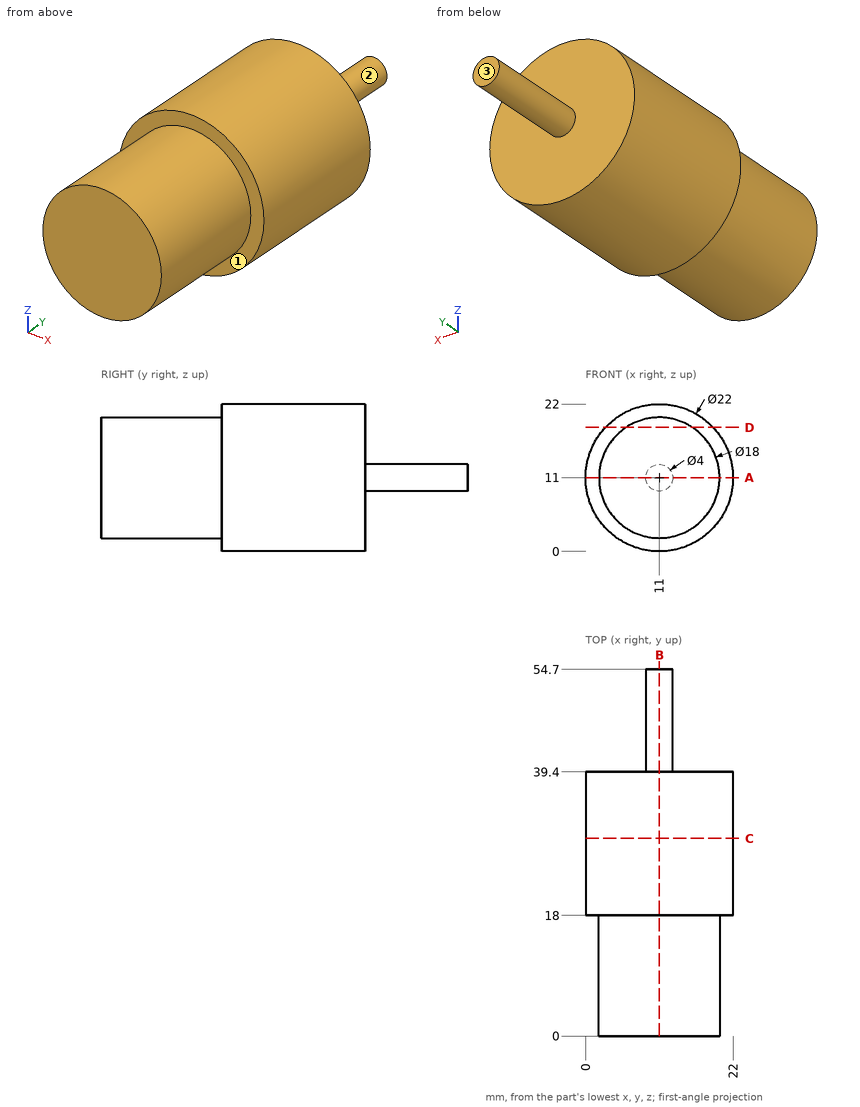
The figure shows three views and two pictorial views of one solid part (mm, origin at its lowest corner). Answer the questions. A direction names the side the tool comes from. Coordinates: 2 decimals unless noted, no trailing zeros. Order: outer loops, then holes, each group sorted by start corner. A loop starts at its lowest first (then second) coordinate and runs counter-clockwise, first axis right, second up.
Q1. Which of the six approach directions +Z, -Z, +X, -X, +Y, -Y give full straight-line access (tool end or side, diameter ignored) to the marked faces 1, 2 and 3?
Q2. A cutting plane is placed at B-B, the plane x = 11. Write down the section's boundary in (y, z).
Q3. A cutting plane is placed at D-D, the plane z = 18.5. Write down the section's boundary in (x, y), and give its area (3 significant figures).
Q4. A cutting plane is placed at A-A, the plane z = 11. Write down the section's boundary in (x, y).
Q5. Given P1, Ø11, axis at x = 9.5, z = 6, coming from the -Y side; P2, Ø1.5, axis at x = 18, y = 28.5, coming from the -Z side; P3, Ø4, axis at x = 18, y = 10, coming from the +Z side; P4, Ø2, axis at x = 7, y = 32.5, coming from the +Z side, each flat-ended and moving along its own axis, determine where each tip first touches the part or whether it passes through.
Q6. A cutting plane is placed at C-C, the plane y = 29.5. Write down the section's boundary in (x, z).
Q7. Consider line 1 (Z direction, x = 11.5, y = 20.5); line 2 (Y direction, x = 8.25, z = 18.25); line 3 (Y direction, x = 16, z = 2.5). Determine where each line is inside the solid, lowest interval first.
Answers follow:
1. face 1: -Y
1. face 2: +Y
1. face 3: +Z, -Z, +X, -X, +Y
2. outline: (0, 2) - (18, 2) - (18, 0) - (39.4, 0) - (39.4, 9) - (54.7, 9) - (54.7, 13) - (39.4, 13) - (39.4, 22) - (18, 22) - (18, 20) - (0, 20) - close
3. outline: (2.95, 18) - (6.03, 18) - (6.03, 0) - (15.97, 0) - (15.97, 18) - (19.05, 18) - (19.05, 39.4) - (2.95, 39.4) - close
3. area: 523 mm2
4. outline: (0, 18) - (2, 18) - (2, 0) - (20, 0) - (20, 18) - (22, 18) - (22, 39.4) - (13, 39.4) - (13, 54.7) - (9, 54.7) - (9, 39.4) - (0, 39.4) - close
5. P1: stops at y = 0
5. P2: stops at z = 1.95
5. P3: stops at z = 18.48
5. P4: stops at z = 21.58
6. outline: circle Ø22 at (11, 11)
7. line 1: z = 0.01 to 21.99
7. line 2: y = 0 to 39.4
7. line 3: y = 18 to 39.4
